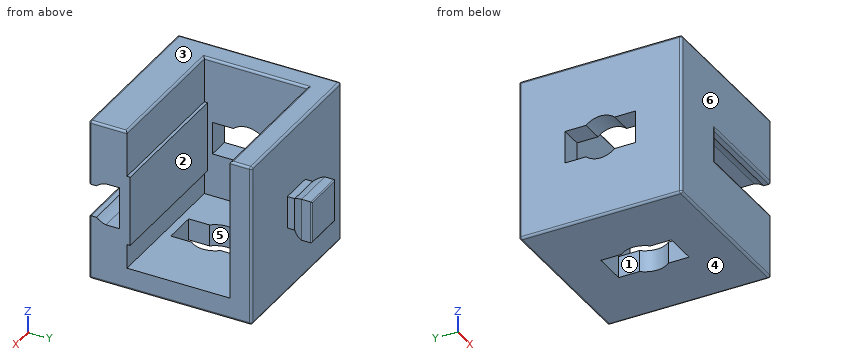
```python
from build123d import *

# Parameters (mm, degrees)
EXTRUDE_1_DEPTH      = 7.5
EXTRUDE_1_DEPTH_BACK = 7.5
SKETCH_1_W           = 15
SKETCH_1_H           = 15
SKETCH_2_W           = 13
SKETCH_2_H           = 9.5
CUT_EXTRUDE_1_DEPTH  = 13
SKETCH_3_W           = 3
SKETCH_3_H           = 3
EXTRUDE_2_DEPTH      = 1
EXTRUDE_3_DEPTH      = 2
EXTRUDE_3_DEPTH_BACK = 2
CUT_EXTRUDE_2_REACH  = 23.256
EXTRUDE_4_REACH      = 26.238
SKETCH_6_W           = 6.5
SKETCH_6_H           = 0.3
CUT_EXTRUDE_3_DEPTH  = 9.45
CUT_EXTRUDE_4_REACH  = 25.054
CUT_EXTRUDE_5_REACH  = 25.054
FILLET_1_R           = 0.1
FILLET_2_R           = 0.2


with BuildPart() as part:
    # Sketch 1 → Extrude 1 (new, two sides: drawn at the far end of the back side and taken through both)
    with BuildSketch(Plane.XY.offset(-EXTRUDE_1_DEPTH_BACK)):
        with Locations((0, 7.5)):
            Rectangle(SKETCH_1_W, SKETCH_1_H)
    extrude(amount=EXTRUDE_1_DEPTH + EXTRUDE_1_DEPTH_BACK)

    # Sketch 2 → Cut-Extrude 1 (cut)
    with BuildSketch(Plane.XY.offset(7.5)):
        with Locations((1, 8.25)):
            Rectangle(SKETCH_2_W, SKETCH_2_H)
    extrude(amount=-CUT_EXTRUDE_1_DEPTH, mode=Mode.SUBTRACT)

    # Sketch 3 → Extrude 2 (add)
    with BuildSketch(Plane(origin=(0, 15, 0), x_dir=(-1, 0, 0), z_dir=(0, 1, 0))):
        Rectangle(SKETCH_3_W, SKETCH_3_H)
    extrude(amount=EXTRUDE_2_DEPTH)

    # Sketch 4 → Extrude 3 (add, two sides: drawn at the far end of the back side and taken through both)
    with BuildSketch(Plane.XY.offset(-EXTRUDE_3_DEPTH_BACK)):
        with BuildLine():
            Line((-1.95, 17.5), (-1.95, 16.555590279))
            ThreePointArc((-1.95, 16.555590279), (-1.780042303, 16.088161527), (-1.5, 15.677124344))
            Line((-1.5, 15.677124344), (1.5, 15.677124344))
            ThreePointArc((1.5, 15.677124344), (1.780042303, 16.088161527), (1.95, 16.555590279))
            Line((1.95, 16.555590279), (1.95, 17.5))
            Line((1.95, 17.5), (-1.95, 17.5))
        make_face()
    extrude(amount=EXTRUDE_3_DEPTH + EXTRUDE_3_DEPTH_BACK)

    # Sketch 5 → Cut-Extrude 2 (cut, up to next)
    with BuildSketch(Plane.ZY.offset(1.95), mode=Mode.PRIVATE) as cut_extrude_2_sk1:
        with BuildLine():
            Line((-1.95, 17.5), (-1.95, 16.555590279))
            ThreePointArc((-1.95, 16.555590279), (-1.780042303, 16.088161527), (-1.5, 15.677124344))
            Line((-1.5, 15.677124344), (-2, 15.677124344))
            Line((-2, 15.677124344), (-2, 17.5))
            Line((-2, 17.5), (-1.95, 17.5))
        make_face()
    cut_extrude_2_tool1 = extrude(cut_extrude_2_sk1.sketch, amount=-CUT_EXTRUDE_2_REACH, mode=Mode.PRIVATE) & part.part
    # Sketch 5 → Cut-Extrude 2 (cut, up to next)
    with BuildSketch(Plane.ZY.offset(1.95), mode=Mode.PRIVATE) as cut_extrude_2_sk2:
        with BuildLine():
            Line((2, 17.5), (2, 15.677124344))
            Line((2, 15.677124344), (1.5, 15.677124344))
            ThreePointArc((1.5, 15.677124344), (1.780042303, 16.088161527), (1.95, 16.555590279))
            Line((1.95, 16.555590279), (1.95, 17.5))
            Line((1.95, 17.5), (2, 17.5))
        make_face()
    cut_extrude_2_tool2 = extrude(cut_extrude_2_sk2.sketch, amount=-CUT_EXTRUDE_2_REACH, mode=Mode.PRIVATE) & part.part
    add(cut_extrude_2_tool1.solids().sort_by_distance((-1.95, 16.175075, -1.873038))[0], mode=Mode.SUBTRACT)
    add(cut_extrude_2_tool2.solids().sort_by_distance((-1.95, 16.175075, 1.873038))[0], mode=Mode.SUBTRACT)

    # Sketch 6 → Extrude 4 (add, up to next)
    with BuildSketch(Plane(origin=(7.5, 0, 0), x_dir=(0, 0, -1), z_dir=(1, 0, 0)), mode=Mode.PRIVATE) as extrude_4_sk1:
        with Locations((0, 3.65)):
            Rectangle(SKETCH_6_W, SKETCH_6_H)
    extrude_4_tool1 = extrude(extrude_4_sk1.sketch, amount=-EXTRUDE_4_REACH, mode=Mode.PRIVATE) - part.part
    add(extrude_4_tool1.solids().sort_by_distance((7.5, 3.65, 0))[0])

    # Sketch 7 → Cut-Extrude 3 (cut)
    with BuildSketch(Plane(origin=(7.5, 0, 0), x_dir=(0, 0, -1), z_dir=(1, 0, 0))):
        with BuildLine():
            Line((-1.5, 0), (1.5, 0))
            Line((1.5, 0), (1.5, 0.677124344))
            ThreePointArc((1.5, 0.677124344), (1.780042303, 1.088161527), (1.95, 1.555590279))
            Line((1.95, 1.555590279), (1.95, 2.8))
            Line((1.95, 2.8), (-1.95, 2.8))
            Line((-1.95, 2.8), (-1.95, 1.555590279))
            ThreePointArc((-1.95, 1.555590279), (-1.780042303, 1.088161527), (-1.5, 0.677124344))
            Line((-1.5, 0.677124344), (-1.5, 0))
        make_face()
    extrude(amount=-CUT_EXTRUDE_3_DEPTH, mode=Mode.SUBTRACT)

    # Sketch 8 → Cut-Extrude 4 (cut, up to next)
    with BuildSketch(Plane.XY.offset(-5.5), mode=Mode.PRIVATE) as cut_extrude_4_sk1:
        with BuildLine():
            Line((-1.5, 8.822875656), (-1.5, 10.75))
            Line((-1.5, 10.75), (1.5, 10.75))
            Line((1.5, 10.75), (1.5, 8.822875656))
            ThreePointArc((1.5, 8.822875656), (2, 7.5), (1.5, 6.177124344))
            Line((1.5, 6.177124344), (1.5, 4.25))
            Line((1.5, 4.25), (-1.5, 4.25))
            Line((-1.5, 4.25), (-1.5, 6.177124344))
            ThreePointArc((-1.5, 6.177124344), (-2, 7.5), (-1.5, 8.822875656))
        make_face()
    cut_extrude_4_tool1 = extrude(cut_extrude_4_sk1.sketch, amount=-CUT_EXTRUDE_4_REACH, mode=Mode.PRIVATE) & part.part
    add(cut_extrude_4_tool1.solids().sort_by_distance((0, 7.5, -5.5))[0], mode=Mode.SUBTRACT)

    # Sketch 9 → Cut-Extrude 5 (cut, up to next)
    with BuildSketch(Plane(origin=(-5.5, 0, 0), x_dir=(0, 0, -1), z_dir=(1, 0, 0)), mode=Mode.PRIVATE) as cut_extrude_5_sk1:
        with BuildLine():
            Line((-1.5, 8.822875656), (-1.5, 10.75))
            Line((-1.5, 10.75), (1.5, 10.75))
            Line((1.5, 10.75), (1.5, 8.822875656))
            ThreePointArc((1.5, 8.822875656), (2, 7.5), (1.5, 6.177124344))
            Line((1.5, 6.177124344), (1.5, 4.25))
            Line((1.5, 4.25), (-1.5, 4.25))
            Line((-1.5, 4.25), (-1.5, 6.177124344))
            ThreePointArc((-1.5, 6.177124344), (-2, 7.5), (-1.5, 8.822875656))
        make_face()
    cut_extrude_5_tool1 = extrude(cut_extrude_5_sk1.sketch, amount=-CUT_EXTRUDE_5_REACH, mode=Mode.PRIVATE) & part.part
    add(cut_extrude_5_tool1.solids().sort_by_distance((-5.5, 7.5, 0))[0], mode=Mode.SUBTRACT)

    # Fillet 1
    fillet_1_edges = [part.edges().sort_by_distance(p)[0] for p in [
        (-1.95, 17.5, 0),
        (1.95, 17.5, 0),
        (0, 17.5, -1.95),
        (0, 17.5, 1.95),
    ]]
    fillet(fillet_1_edges, radius=FILLET_1_R)

    # Fillet 2
    fillet_2_edges = [part.edges().sort_by_distance(p)[0] for p in [
        (7.5, 7.5, -7.5),
        (7.5, 0, 4.5),
        (-7.5, 7.5, 7.5),
        (-1.95, 0, 0),
        (2.775, 0, -1.5),
        (2.775, 0, 1.5),
        (0, 0, 7.5),
        (0, 15, -7.5),
        (7.5, 1.75, 7.5),
        (0, 15, 7.5),
        (7.5, 14, 7.5),
        (-5.5, 8.25, 7.5),
        (1, 3.5, 7.5),
        (1, 13, 7.5),
        (-7.5, 7.5, -7.5),
        (0, 0, -7.5),
        (-7.5, 15, 0),
        (7.5, 15, 0),
        (7.5, 0, -4.5),
        (-7.5, 0, 0),
    ]]
    fillet(fillet_2_edges, radius=FILLET_2_R)


solid = part.part
```
The listing builds one solid part. Answer for the finished solid, in the listing's coordinates (mm). Face numbers are marked on the shaded views. A direction names the side the tool comes from. Give positions to 0.01 mm unless a question says otherwise; leave off trailing zeros. Loops run counter-clockwise (first coordinate to the right, second up) from the corner with the lowest first, then second, coordinate; pieces in that order, holes last. Notation, with made-up numbers: (-0.75, 83) - (53.25, 83) arc R36 ccw to (53.25, 120) - close; hole circle Ø11 at (26.5, 19.25). An arc over 180 degrees is marked (long way). Return JSON: item names as keys, results as strings. Group by question number.
1. Find section C-C (x = -6). Write down the section's boundary in (y, z).
2. Find section A-A (z = -1). Write down the section's boundary in (x, y).
3. Find section B-B (y = 10.5). Write down the section's boundary in (x, z), then the cut area to 3 significant figures.
4. Given pin 1 Ø2 at (x, z) = (0, 4.5) entering from +Y; pin 2 Ø0.9 at (x, y) = (1, 17) entering from +Z; pin 3 Ø1.5 at (x, y) = (-4, 10) entering from +Z, each flat-ended and moving along its own axis, determine where each tip first touches the part or whether it passes through.
5. Determine the mould class of the marked faces 4, 5 and 6 for opening direction Y: pulls with the +Y half, pulls with the -Y half, needs draft (parallel to the pull), parting line crosses it, or undercut.
6. Find section D-D (x = -2.75). Write down the section's boundary in (y, z).
7. Which of the six approach directions +Z, -Z, +X, -X, +Y, -Y give full straight-line access (tool end or side, diameter ignored) to the marked faces 1, 2 and 3?
8. Straight lines are drawn through the part: line 1 (Y direction, x = 4.75, z = 5.25); line 2 (Z direction, x = -0.5, y = 2.5); line 3 (Y direction, x = -1, z = 2.75). For each, find the intervals that lie inside material, in ascending order. Write a range as [from, to].
Verdict:
{
 "1": {"outline": "(0, -7.3) arc R0.2 ccw to (0.2, -7.5) - (14.8, -7.5) arc R0.2 ccw to (15, -7.3) - (15, 7.3) arc R0.2 ccw to (14.8, 7.5) - (0.2, 7.5) arc R0.2 ccw to (0, 7.3) - close; hole (4.25, -1.5) - (6.18, -1.5) arc R2 ccw to (8.82, -1.5) - (10.75, -1.5) - (10.75, 1.5) - (8.82, 1.5) arc R2 ccw to (6.18, 1.5) - (4.25, 1.5) - close"},
 "2": {"outline": "(-7.5, 0.2) arc R0.2 ccw to (-7.3, 0) - (-2.15, 0) arc R0.2 ccw to (-1.95, 0.2) - (-1.95, 2.8) - (7.5, 2.8) - (7.5, 3.8) - (-5.5, 3.8) - (-5.5, 4.25) - (-7.5, 4.25) - close; (-7.5, 10.75) - (-5.5, 10.75) - (-5.5, 13) - (7.5, 13) - (7.5, 14.8) arc R0.2 ccw to (7.3, 15) - (1.5, 15) - (1.5, 15.68) arc R2 ccw to (1.95, 16.56) - (1.95, 17.4) arc R0.1 ccw to (1.85, 17.5) - (-1.85, 17.5) arc R0.1 ccw to (-1.95, 17.4) - (-1.95, 16.56) arc R2 ccw to (-1.5, 15.68) - (-1.5, 15) - (-7.3, 15) arc R0.2 ccw to (-7.5, 14.8) - close"},
 "3": {"outline": "(-7.5, -7.3) arc R0.2 ccw to (-7.3, -7.5) - (-1.5, -7.5) - (-1.5, -5.5) - (-5.5, -5.5) - (-5.5, -1.5) - (-7.5, -1.5) - close; (-7.5, 1.5) - (-5.5, 1.5) - (-5.5, 7.3) arc R0.2 ccw to (-5.7, 7.5) - (-7.3, 7.5) arc R0.2 ccw to (-7.5, 7.3) - close; (1.5, -7.5) - (7.3, -7.5) arc R0.2 ccw to (7.5, -7.3) - (7.5, -5.5) - (1.5, -5.5) - close", "area": "44.0 mm^2"},
 "4": {"pin 1": "stops at y = 15", "pin 2": "stops at z = 1.95", "pin 3": "stops at z = -5.5"},
 "5": {"face 4": "needs draft", "face 5": "undercut", "face 6": "pulls with the -Y half"},
 "6": {"outline": "(0, -7.3) arc R0.2 ccw to (0.2, -7.5) - (14.8, -7.5) arc R0.2 ccw to (15, -7.3) - (15, 7.3) arc R0.2 ccw to (14.8, 7.5) - (13.2, 7.5) arc R0.2 ccw to (13, 7.3) - (13, -5.5) - (3.5, -5.5) - (3.5, -3.25) - (3.8, -3.25) - (3.8, 3.25) - (3.5, 3.25) - (3.5, 7.3) arc R0.2 ccw to (3.3, 7.5) - (0.2, 7.5) arc R0.2 ccw to (0, 7.3) - close"},
 "7": {"face 1": "+Z, -Z", "face 2": "+Z, +X", "face 3": "+Z, +X, -X, +Y, -Y"},
 "8": {"line 1": "y = [0, 3.5], [13, 15]", "line 2": "z = [-7.5, -1.95], [1.95, 7.5]", "line 3": "y = [0, 3.8], [13, 15]"}
}
